Design review of the part built by this model. Coordinates are the model's own, in mm. Coordinates: 2 decimals unless noted, no trailing zeros. Loops run counter-clockwise (first coordinate to the right, second up) from the corner with the lowest first, then second, coordinate; pieces in that order, holes last. Notation, with made-up numbers: (11, 69) -> (58, 69) arc R33 cw to (58, 97) -> close; hole circle Ø1 at (37.5, 60). An arc over 180 degrees is marked (long way). One line per item, written item: value. Start each with the question number.
1. Insertion check: pin 1 (6.5 mm diameter, centred on x = -20.98, y = 84, fed in from +Z); pin 2 (4.5 mm diameter, centred on x = 39.02, y = -84, fed in from +Z). Each pin has a flat end and moves straight along its axis. Give the tip position at first contact, or say it passes through.
2. For probe 1 along Y at (x, z) = (-20.5, 4.6); probe 2 along Y at (x, z) = (40, 1.6), list the stretches that pass through material, from the lowest coordinate up.
3. Add section A-A on y = 84. Write out the cut boundary in (x, z).
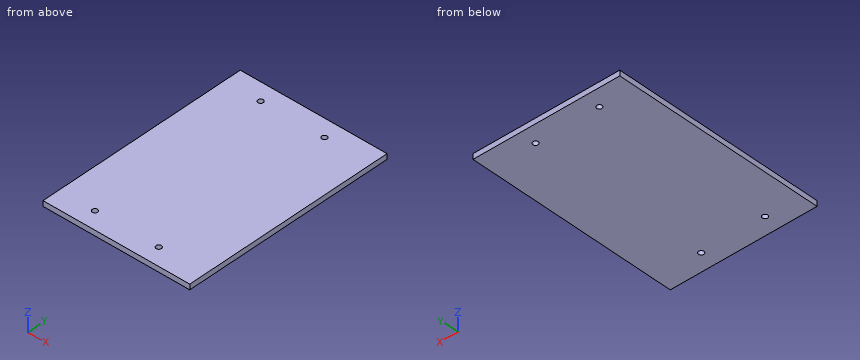
```python
from build123d import *

# Parameters (mm, degrees)
ESQUISSE1_W             = 110
ESQUISSE1_H             = 200
BOSS_EXTRU_1_DEPTH      = 5
ESQUISSE28_R            = 2.5
ENL_V_MAT_EXTRU_1_DEPTH = 115.236596588
ESQUISSE29_W            = 5
ESQUISSE29_H            = 200
BOSS_EXTRU_2_DEPTH      = 28


with BuildPart() as part:
    # Esquisse1 → Boss.-Extru.1 (new body)
    with BuildSketch(Plane.XY):
        Rectangle(ESQUISSE1_W, ESQUISSE1_H)
    extrude(amount=BOSS_EXTRU_1_DEPTH)

    # Esquisse28 → Enlèv. mat.-Extru.1 (cut, through all)
    with BuildSketch(Plane(origin=(0, 0, 0), x_dir=(-1, 0, 0), z_dir=(0, 0, -1))):
        with Locations((20.980762114, -84)):
            Circle(ESQUISSE28_R)
        with Locations((-39.019237886, -84)):
            Circle(ESQUISSE28_R)
        with Locations((20.980762114, 84)):
            Circle(ESQUISSE28_R)
        with Locations((-39.019237886, 84)):
            Circle(ESQUISSE28_R)
    extrude(amount=-ENL_V_MAT_EXTRU_1_DEPTH, mode=Mode.SUBTRACT)

    # Esquisse29 → Boss.-Extru.2 (add)
    with BuildSketch(Plane(origin=(55, 0, 0), x_dir=(0, 0, -1), z_dir=(1, 0, 0))):
        with Locations((-2.5, 0)):
            Rectangle(ESQUISSE29_W, ESQUISSE29_H)
    extrude(amount=BOSS_EXTRU_2_DEPTH)


solid = part.part
```
Worked answers:
1. pin 1: stops at z = 5
1. pin 2: passes through
2. probe 1: y = -100 to -86.45, -81.55 to 81.55, 86.45 to 100
2. probe 2: y = -100 to -86.3, -81.7 to 81.7, 86.3 to 100
3. outline: (-55, 0) -> (-23.48, 0) -> (-23.48, 5) -> (-55, 5) -> close; (-18.48, 0) -> (36.52, 0) -> (36.52, 5) -> (-18.48, 5) -> close; (41.52, 0) -> (83, 0) -> (83, 5) -> (41.52, 5) -> close
